Verification items for the finished model (mm, model axes). A direction names the side the tool comes from. Round coordinates to 2 decimals unless told otherwise and drop trailing zeros. Loops run counter-clockwise (first coordinate to the right, second up) from the corner with the lowest first, then second, coordinate; pieces in that order, holes last. Notation, with made-up numbers: M 21,65 L 55,65 A28 cw 55,96 Z; hole C 59.5,-31 d10. An arc over 180 degrees is marked long. One line per item, written item: value.
from build123d import *

# Parameters (mm, degrees)
SKETCH5_W           = 26
SKETCH5_H           = 26
BOSS_EXTRUDE1_DEPTH = 10
SKETCH4_R           = 10.75
CUT_EXTRUDE1_DEPTH  = 4
SKETCH6_W           = 10
SKETCH6_H           = 3.483566845
CUT_EXTRUDE2_DEPTH  = 4
LPATTERN1_COUNT     = 6
LPATTERN1_PITCH     = 26
SKETCH7_W           = 10
SKETCH7_H           = 4
CUT_EXTRUDE3_DEPTH  = 131
FILLET1_R           = 2
SKETCH9_W           = 8
SKETCH9_H           = 3
CUT_EXTRUDE4_DEPTH  = 3


with BuildPart() as part:
    # Sketch5 → Boss-Extrude1 (new body)
    with BuildSketch(Plane(origin=(0, 0, 0), x_dir=(1, 0, 0), z_dir=(0, 1, 0))):
        Rectangle(SKETCH5_W, SKETCH5_H)
    boss_extrude1 = extrude(amount=-BOSS_EXTRUDE1_DEPTH)

    # Sketch4 → Cut-Extrude1 (cut)
    with BuildSketch(Plane(origin=(0, 0, 0), x_dir=(1, 0, 0), z_dir=(0, 1, 0))):
        Circle(SKETCH4_R)
    cut_extrude1 = extrude(amount=-CUT_EXTRUDE1_DEPTH, mode=Mode.SUBTRACT)

    # Sketch6 → Cut-Extrude2 (cut)
    with BuildSketch(Plane(origin=(0, 0, 0), x_dir=(1, 0, 0), z_dir=(0, 1, 0))):
        with Locations((0, 11.258216578)):
            Rectangle(SKETCH6_W, SKETCH6_H)
    cut_extrude2 = extrude(amount=-CUT_EXTRUDE2_DEPTH, mode=Mode.SUBTRACT)

    # LPattern1: Boss-Extrude1, Cut-Extrude1, Cut-Extrude2 ×6
    with Locations(*[(0, 0, -i * LPATTERN1_PITCH) for i in range(1, LPATTERN1_COUNT)]):
        add(boss_extrude1)
        add(cut_extrude1, mode=Mode.SUBTRACT)
        add(cut_extrude2, mode=Mode.SUBTRACT)

    # Sketch7 → Cut-Extrude3 (cut, through all)
    with BuildSketch(Plane.XY.offset(-13)):
        with Locations((0, -2)):
            Rectangle(SKETCH7_W, SKETCH7_H)
    extrude(amount=-CUT_EXTRUDE3_DEPTH, mode=Mode.SUBTRACT)

    # Fillet1
    fillet1_edges = [part.edges().sort_by_distance(p)[0] for p in [
        (13, -5, -143),
        (-13, -5, -143),
        (13, -5, 13),
        (-13, -5, 13),
    ]]
    fillet(fillet1_edges, radius=FILLET1_R)

    # Sketch9 → Cut-Extrude4 (cut)
    with BuildSketch(Plane(origin=(0, 0, -143), x_dir=(-1, 0, 0), z_dir=(0, 0, -1))):
        with Locations((0, -7)):
            Rectangle(SKETCH9_W, SKETCH9_H)
    extrude(amount=-CUT_EXTRUDE4_DEPTH, mode=Mode.SUBTRACT)


solid = part.part
(1) Tool access check on faces 5 (the face through (-10.75, -1.97, -78.16)), 6 (the face through (5, -2, -117)), 7 (the face through (0, -5.5, -142)). Record the directions out of +Z, -Z, +X, -X, +Y, -Y that give a thin tool (end or side, any length) a straight path to the whole face; none if there is none.
Completed:
face 5: +Y
face 6: -Z, +Y
face 7: -Z
(2) Sectioned sample at D-D on z = -41. Enter the section's corners in (x, y), and give its area (3 significant figures).
Completed:
outline: M -13,-10 L 13,-10 L 13,0 L 5,0 L 5,-4 L -5,-4 L -5,0 L -13,0 Z
area: 220 mm^2
(3) Depth check by flat-ended pin: pin 1 Ø4 at (y, z) = (-1.5, -142) entering from +X; pin 2 Ø0.9 at (x, y) = (-1, -7.5) entering from -Z. Enter the tip coordinate at first touch or a pass-through.
Completed:
pin 1: stops at x = 13
pin 2: stops at z = -140
(4) Mould release check, pull along X, two halves, no side actions. Record for faces 1 (the face through (13, -5, -64)), 2 (the face through (5, -2, -13)), 3 (the face through (-6, 0, -66)), 4 (the face through (10.75, -1.97, -25.84)): +X half, -X half, draft (parallel to the pull), parting line (faces both ways), or undercut.
Completed:
face 1: +X half
face 2: undercut
face 3: draft
face 4: undercut
(5) Sectioned sample at C-C on x = 0. Enter the section's corners in (y, z).
Completed:
outline: M -10,-143 L -8.5,-143 L -8.5,-140 L -5.5,-140 L -5.5,-143 L -4,-143 L -4,10.75 L 0,10.75 L 0,13 L -10,13 Z
(6) Sectioned sample at B-B on z = 0. Enter the section's corners in (x, y).
Completed:
outline: M -13,-10 L 13,-10 L 13,0 L 10.75,0 L 10.75,-4 L -10.75,-4 L -10.75,0 L -13,0 Z
(7) Thickness scan on L1, parallel to X at y = -1.2, z = 0; L2, parallel to Y at x = -5.75, z = -71.5; L3, parallel to Z at x = 0, y = -1.3. Record the ranges inside material, lowest first. Write a range as from..to.
Completed:
L1: x = -13..-10.75, 10.75..13
L2: y = -10..-4
L3: z = 10.75..13
